Could you check a few things on this model? Use its own coordinates, in mm. A direction names the side the tool comes from. Round coordinates to 2 decimals unless told otherwise and drop trailing zeros. Write each loop counter-clockwise with the first axis right and the second up, starting at its lowest first coordinate (ties: lowest second). Pieces come first, ordered by that corner, then holes. Notation, with made-up numbers: (-12.75, 66.25) -> (11.25, 66.25) arc R14 cw to (11.25, 73.25) -> close; hole circle Ø3 at (44, 63). An arc over 180 degrees is marked (long way). Return JSON: item names as keys, results as strings.
from build123d import *

# Parameters (mm, degrees)
F0_W     = 16
F0_H     = 20
F0_W_2   = 14
F0_H_2   = 17
F1_DEPTH = 4
F2_R     = 4
F3_DEPTH = 16
F4_R     = 3
F5_DEPTH = 16


with BuildPart() as f1:
    # F0 (on Top) → F1 (new body)
    with BuildSketch(Plane.XY):
        with Locations((-4.000824, -1.813023)):
            Rectangle(F0_W, F0_H)
        with Locations((-3.993993, -1.764975)):
            Rectangle(F0_W_2, F0_H_2, mode=Mode.SUBTRACT)
    extrude(amount=-F1_DEPTH)

    # F2 (on face) → F3 (join)
    with BuildSketch(Plane(origin=(-12.000824, 0, 0), x_dir=(0, -1, 0), z_dir=(-1, 0, 0))):
        with Locations((-11.607357, -2)):
            Circle(F2_R)
        with Locations((15.161447, -2)):
            Circle(F2_R)
    extrude(amount=-F3_DEPTH)

    # F4 (on face) → F5 (cut)
    with BuildSketch(Plane.YZ.offset(3.999176)):
        with Locations((-15.161447, -2)):
            Circle(F4_R)
        with Locations((11.607357, -2)):
            Circle(F4_R)
    extrude(amount=-F5_DEPTH, mode=Mode.SUBTRACT)


solid = f1.part
1) Thinking about a two-plate mould opening in Y: for faces 1 (the face through (3.006, -2, -2)), 2 (the face through (3.999, -2, -2)), which applies, pulls with the +Y half, pulls with the -Y half, needs draft (parallel to the pull), parting line crosses it, or undercut?
Return value:
{"face 1": "undercut", "face 2": "needs draft"}
2) Will these pins go through, and if not, where does the flat tip stop? pin 1 Ø4 at (x, y) = (-0.5, 9) entering from -Z; pin 2 Ø2 at (x, z) = (-10, -5) entering from -Y.
Return value:
{"pin 1": "z = -5.95", "pin 2": "y = -18.63"}
3) For faces 3 (the face through (-4, -10.265, -2)), 4 (the face through (-12.001, -2, -2)), 5 (the face through (-11.15, -1.73, -4)), 6 (the face through (-11.15, -1.73, 0)), 7 (the face through (-3.9, 14.4, -3.1)), which set-ups out of +Z, -Z, +X, -X, +Y, -Y let a thin tool reach every point of the face, with its end or its side?
Return value:
{"face 3": "+Z, -Z", "face 4": "+Z, -Z, -X, +Y, -Y", "face 5": "-Z, +X, -X", "face 6": "+Z, +X, -X", "face 7": "+X, -X"}
4) If I drill on probe 1 along Y at (x, z) = (-10, -0.75); probe 2 along Y at (x, z) = (0, -2.25); probe 3 along X at (y, z) = (5, -2.5), over which ranges is the centre line in solid material (lowest first)? Write a range as [from, to].
Return value:
{"probe 1": "[-18.96, -17.89], [-12.43, -10.26], [6.74, 8.88], [14.33, 15.41]", "probe 2": "[-19.15, -18.15], [-12.17, -10.26], [6.74, 8.62], [14.6, 15.6]", "probe 3": "[-12, -10.99], [3.01, 4]"}
5) I want a section at B-B, the plane z = -2. Please give me the cut outline in (x, y).
Return value:
{"outline": "(-12, -19.16) -> (4, -19.16) -> (4, -18.16) -> (-12, -18.16) -> close; (-12, -12.16) -> (4, -12.16) -> (4, 8.61) -> (-12, 8.61) -> close; (-12, 14.61) -> (4, 14.61) -> (4, 15.61) -> (-12, 15.61) -> close; hole (-10.99, -10.26) -> (3.01, -10.26) -> (3.01, 6.74) -> (-10.99, 6.74) -> close"}
6) I want a section at C-C, the plane y = 0. Please give me the cut outline in (x, z), and give its area (3 significant figures).
Return value:
{"outline": "(-12, -4) -> (-10.99, -4) -> (-10.99, 0) -> (-12, 0) -> close; (3.01, -4) -> (4, -4) -> (4, 0) -> (3.01, 0) -> close", "area": "8.00 mm²"}
7) I want a section at D-D, the plane z = 1.5. Please give me the cut outline in (x, y), and give its area (3 significant figures).
Return value:
{"outline": "(-12, -17.1) -> (4, -17.1) -> (4, -13.22) -> (-12, -13.22) -> close; (-12, 9.67) -> (4, 9.67) -> (4, 13.54) -> (-12, 13.54) -> close", "area": "124 mm²"}
8) I want a section at A-A, the plane x = -3.25. Please give me the cut outline in (y, z), and give its area (3 significant figures).
Return value:
{"outline": "(-11.7, -4) -> (-10.26, -4) -> (-10.26, 0) -> (-11.7, 0) arc R4 ccw (long way) to start; (6.74, -4) -> (8.14, -4) arc R4 ccw (long way) to (8.14, 0) -> (6.74, 0) -> close; hole circle Ø6 at (-15.16, -2); hole circle Ø6 at (11.61, -2)", "area": "52.4 mm²"}
